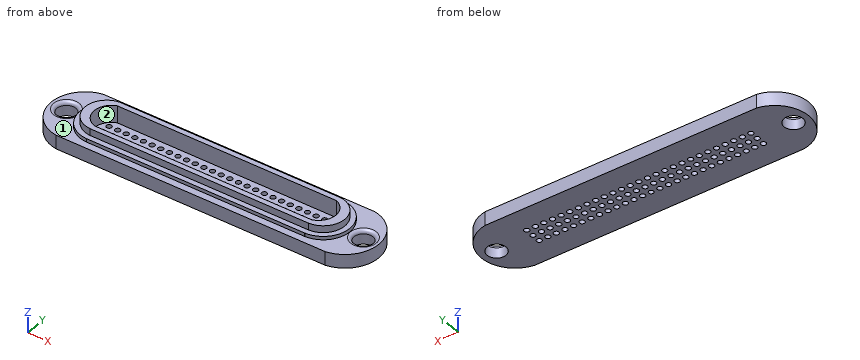
from build123d import *

# Parameters (mm, degrees)
F0_R     = 2.75
F1_DEPTH = 4
F2_DEPTH = 5
F3_DEPTH = 7
F4_DEPTH = 2
F5_R     = 0.75
F5_R_2   = 0.7
F6_DEPTH = 25
F7_R     = 1


with BuildPart() as f1:
    # F0 (on Top) → F1 (new body)
    with BuildSketch(Plane.XY):
        with BuildLine():
            Line((-38.977494, -9.75), (0, -9.75))
            Line((0, -9.75), (38.977494, -9.75))
            ThreePointArc((38.977494, -9.75), (47.498043, -0.167837), (39.370675, 9.75))
            Line((39.370675, 9.75), (0, 9.75))
            Line((0, 9.75), (-39.370675, 9.75))
            ThreePointArc((-39.370675, 9.75), (-47.498043, -0.167837), (-38.977494, -9.75))
        make_face()
        with Locations((-43, 0)):
            Circle(F0_R, mode=Mode.SUBTRACT)
        with BuildLine():
            ThreePointArc((-31.644462, -7.748965), (-39.122501, -0.217996), (-32.104186, 7.743147))
            Line((-32.104186, 7.743147), (-31.961884, 7.75))
            Line((-31.961884, 7.75), (0, 7.75))
            Line((0, 7.75), (31.961884, 7.75))
            Line((31.961884, 7.75), (32.104186, 7.743147))
            ThreePointArc((32.104186, 7.743147), (39.122501, -0.217996), (31.644462, -7.748965))
            Line((31.644462, -7.748965), (31.587565, -7.75))
            Line((31.587565, -7.75), (0.328864, -7.75))
            Line((0.328864, -7.75), (-0.328864, -7.75))
            Line((-0.328864, -7.75), (-31.587565, -7.75))
            Line((-31.587565, -7.75), (-31.644462, -7.748965))
        make_face(mode=Mode.SUBTRACT)
        with Locations((43, 0)):
            Circle(F0_R, mode=Mode.SUBTRACT)
    extrude(amount=F1_DEPTH)

    # F0 (on Top) → F2 (join)
    with BuildSketch(Plane.XY):
        with BuildLine():
            Line((-31.961884, 7.75), (-32.104186, 7.743147))
            ThreePointArc((-32.104186, 7.743147), (-39.122501, -0.217996), (-31.644462, -7.748965))
            Line((-31.644462, -7.748965), (-31.587565, -7.75))
            Line((-31.587565, -7.75), (-0.328864, -7.75))
            Line((-0.328864, -7.75), (0.328864, -7.75))
            Line((0.328864, -7.75), (31.587565, -7.75))
            Line((31.587565, -7.75), (31.644462, -7.748965))
            ThreePointArc((31.644462, -7.748965), (39.122501, -0.217996), (32.104186, 7.743147))
            Line((32.104186, 7.743147), (31.961884, 7.75))
            Line((31.961884, 7.75), (0, 7.75))
            Line((0, 7.75), (-31.961884, 7.75))
        make_face()
        with BuildLine():
            Line((31.587565, -6.25), (-0.328864, -6.25))
            Line((-0.328864, -6.25), (-5.279422, -6.25))
            Line((-5.279422, -6.25), (-31.588749, -6.25))
            ThreePointArc((-31.588749, -6.25), (-37.623142, -0.174144), (-31.960962, 6.25))
            Line((-31.960962, 6.25), (0, 6.25))
            Line((0, 6.25), (31.961884, 6.25))
            ThreePointArc((31.961884, 6.25), (37.62311, -0.175133), (31.587565, -6.25))
        make_face(mode=Mode.SUBTRACT)
    extrude(amount=F2_DEPTH)

    # F0 (on Top) → F3 (join)
    with BuildSketch(Plane.XY):
        with BuildLine():
            Line((-5.279422, -6.25), (-0.328864, -6.25))
            Line((-0.328864, -6.25), (31.587565, -6.25))
            ThreePointArc((31.587565, -6.25), (37.62311, -0.175133), (31.961884, 6.25))
            Line((31.961884, 6.25), (0, 6.25))
            Line((0, 6.25), (-31.960962, 6.25))
            ThreePointArc((-31.960962, 6.25), (-37.623142, -0.174144), (-31.588749, -6.25))
            Line((-31.588749, -6.25), (-5.279422, -6.25))
        make_face()
        with BuildLine():
            Line((31.389172, -4.75), (-0.328864, -4.75))
            Line((-0.328864, -4.75), (-5.279422, -4.75))
            Line((-5.279422, -4.75), (-31.389172, -4.75))
            ThreePointArc((-31.389172, -4.75), (-34.997071, -0.117987), (-31.714512, 4.75))
            Line((-31.714512, 4.75), (0, 4.75))
            Line((0, 4.75), (31.714512, 4.75))
            ThreePointArc((31.714512, 4.75), (34.997071, -0.117987), (31.389172, -4.75))
        make_face(mode=Mode.SUBTRACT)
    extrude(amount=F3_DEPTH)

    # F0 (on Top) → F4 (join)
    with BuildSketch(Plane.XY):
        with BuildLine():
            Line((-5.279422, -4.75), (-0.328864, -4.75))
            Line((-0.328864, -4.75), (31.389172, -4.75))
            ThreePointArc((31.389172, -4.75), (34.997071, -0.117987), (31.714512, 4.75))
            Line((31.714512, 4.75), (0, 4.75))
            Line((0, 4.75), (-31.714512, 4.75))
            ThreePointArc((-31.714512, 4.75), (-34.997071, -0.117987), (-31.389172, -4.75))
            Line((-31.389172, -4.75), (-5.279422, -4.75))
        make_face()
    extrude(amount=F4_DEPTH)

    # F5 (on face) → F6 (cut)
    with BuildSketch(Plane.XY.offset(2)):
        with BuildLine():
            ThreePointArc((0, 0.75), (-0.75, 0), (0, -0.75))
            ThreePointArc((0, -0.75), (0.75, 0), (0, 0.75))
        make_face()
        with BuildLine():
            ThreePointArc((0, 3.25), (-0.75, 2.5), (0, 1.75))
            ThreePointArc((0, 1.75), (0.75, 2.5), (0, 3.25))
        make_face()
        with Locations((2.5, 0)):
            Circle(F5_R)
        with Locations((2.5, 2.5)):
            Circle(F5_R)
        with Locations((5, 0)):
            Circle(F5_R)
        with Locations((5, 2.5)):
            Circle(F5_R)
        with Locations((7.5, 0)):
            Circle(F5_R)
        with Locations((7.5, 2.5)):
            Circle(F5_R)
        with Locations((10, 0)):
            Circle(F5_R)
        with Locations((10, 2.5)):
            Circle(F5_R)
        with Locations((12.5, 0)):
            Circle(F5_R)
        with Locations((12.5, 2.5)):
            Circle(F5_R)
        with Locations((15, 0)):
            Circle(F5_R)
        with Locations((15, 2.5)):
            Circle(F5_R)
        with Locations((17.5, 0)):
            Circle(F5_R)
        with Locations((17.5, 2.5)):
            Circle(F5_R)
        with Locations((20, 0)):
            Circle(F5_R)
        with Locations((20, 2.5)):
            Circle(F5_R)
        with Locations((22.5, 0)):
            Circle(F5_R)
        with Locations((22.5, 2.5)):
            Circle(F5_R)
        with Locations((25, 0)):
            Circle(F5_R)
        with Locations((25, 2.5)):
            Circle(F5_R)
        with Locations((27.5, 0)):
            Circle(F5_R)
        with Locations((27.5, 2.5)):
            Circle(F5_R)
        with Locations((2.5, -2.5)):
            Circle(F5_R)
        with Locations((5, -2.5)):
            Circle(F5_R)
        with Locations((7.5, -2.5)):
            Circle(F5_R)
        with Locations((10, -2.5)):
            Circle(F5_R)
        with Locations((12.5, -2.5)):
            Circle(F5_R)
        with Locations((15, -2.5)):
            Circle(F5_R)
        with Locations((17.5, -2.5)):
            Circle(F5_R)
        with Locations((20, -2.5)):
            Circle(F5_R)
        with Locations((22.5, -2.5)):
            Circle(F5_R)
        with Locations((25, -2.5)):
            Circle(F5_R)
        with Locations((27.5, -2.5)):
            Circle(F5_R)
        with Locations((-12.5, 0)):
            Circle(F5_R)
        with Locations((-17.5, 0)):
            Circle(F5_R)
        with Locations((-7.5, 0)):
            Circle(F5_R)
        with Locations((-5, 0)):
            Circle(F5_R)
        with Locations((-15, 0)):
            Circle(F5_R)
        with Locations((-20, 0)):
            Circle(F5_R)
        with Locations((-10, 0)):
            Circle(F5_R)
        with Locations((-12.5, 2.5)):
            Circle(F5_R)
        with Locations((-10, 2.5)):
            Circle(F5_R)
        with Locations((-7.5, 2.5)):
            Circle(F5_R)
        with Locations((-5, 2.5)):
            Circle(F5_R)
        with Locations((-2.5, 0)):
            Circle(F5_R)
        with Locations((-2.5, 2.5)):
            Circle(F5_R)
        with Locations((-17.5, 2.5)):
            Circle(F5_R)
        with Locations((-15, 2.5)):
            Circle(F5_R)
        with Locations((-20, 2.5)):
            Circle(F5_R)
        with Locations((-27.5, 0)):
            Circle(F5_R)
        with Locations((-22.5, 0)):
            Circle(F5_R)
        with Locations((-25, 0)):
            Circle(F5_R)
        with Locations((-27.5, -2.5)):
            Circle(F5_R)
        with Locations((-25, 2.5)):
            Circle(F5_R)
        with Locations((-22.5, 2.5)):
            Circle(F5_R)
        with Locations((-17.5, -2.5)):
            Circle(F5_R)
        with Locations((-27.5, 2.5)):
            Circle(F5_R)
        with Locations((-20, -2.5)):
            Circle(F5_R)
        with Locations((-22.5, -2.5)):
            Circle(F5_R)
        with Locations((-25, -2.5)):
            Circle(F5_R)
        with Locations((-2.5, -2.5)):
            Circle(F5_R)
        with Locations((-5, -2.5)):
            Circle(F5_R)
        with Locations((-7.5, -2.5)):
            Circle(F5_R)
        with Locations((-10, -2.5)):
            Circle(F5_R)
        with Locations((-12.5, -2.5)):
            Circle(F5_R)
        with Locations((-15, -2.5)):
            Circle(F5_R)
        with Locations((0.020794, -2.485011)):
            Circle(F5_R_2)
        with Locations((-29.956931, 0.036661)):
            Circle(F5_R)
        with Locations((29.956931, 0.036661)):
            Circle(F5_R)
        with Locations((29.949998, 2.5)):
            Circle(F5_R)
        with Locations((32.449998, 2.5)):
            Circle(F5_R)
        with Locations((29.949998, -2.5)):
            Circle(F5_R)
        with Locations((32.449998, 0)):
            Circle(F5_R)
        with Locations((32.449998, -2.5)):
            Circle(F5_R)
        with Locations((-32.466013, 0.00955)):
            Circle(F5_R)
        with Locations((-32.466013, -2.49045)):
            Circle(F5_R)
        with Locations((-29.966013, 2.50955)):
            Circle(F5_R)
        with Locations((-32.466013, 2.50955)):
            Circle(F5_R)
        with Locations((-29.966013, -2.49045)):
            Circle(F5_R)
    extrude(amount=-F6_DEPTH, mode=Mode.SUBTRACT)

    # F7
    f7_edges = [f1.edges().sort_by_distance(p)[0] for p in [
        (-45.75, 0, 4),
        (40.25, 0, 4),
    ]]
    fillet(f7_edges, radius=F7_R)


solid = f1.part
Verification items for the finished model (mm, model axes). Face numbers are marked on the shaded views. Give positions to 0.01 mm unless a question says otherwise; leave off trailing zeros. Loops run counter-clockwise (first coordinate to the right, second up) from the corner with the lowest first, then second, coordinate; pieces in that order, holes last.
1) Draft check along Y on the marked faces 1 and 2. Enter one of: pulls with the +Y half, pulls with the -Y half, needs draft (parallel to the pull), parting line crosses it, or undercut.
2) Thickness scan on line 1 along Y through (x, z) = (25, 0.4); line 2 along Y through (x, z) = (30, 3.5); line 3 along Z through (x, y) = (-16.5, -3.5). Record the ranges inside material, lowest first.
3) Depth check by flat-ended pin: pin 1 Ø2 at (x, y) = (-32.47, 0.01) entering from +Z; pin 2 Ø4 at (y, z) = (-5, 3.5) entering from +X. Enter the tip coordinate at first touch or a pass-through.
4) Sectioned sample at A-A, the plane x = -43. Enter the section's corners in (y, z).
Answers:
1. face 1: needs draft
1. face 2: undercut
2. line 1: y = -9.75 to -3.25, -1.75 to -0.75, 0.75 to 1.75, 3.25 to 9.75
2. line 2: y = -9.75 to -4.75, 4.75 to 9.75
2. line 3: z = 0 to 2
3. pin 1: stops at z = 2
3. pin 2: stops at x = 47.02
4. outline: (-8.25, 0) - (-2.75, 0) - (-2.75, 3) arc R1 ccw to (-3.75, 4) - (-8.25, 4) - close; (2.75, 0) - (8.31, 0) - (8.31, 4) - (3.75, 4) arc R1 ccw to (2.75, 3) - close
